Here's how the part is built. I have some questions about the finished solid (model axes, mm). Face numbers are marked on the shaded views. A direction names the side the tool comes from. Give positions to 0.01 mm unless a question says otherwise; leave off trailing zeros. Write each loop counter-clockwise with the first axis right and the second up, starting at its lowest first coordinate (ties: lowest second). Pieces come first, ordered by that corner, then holes. Notation, with made-up numbers: (56, 1) -> (74, 1) arc R22 cw to (74, 12) -> close; hole circle Ø7 at (49.5, -5). An arc over 180 degrees is marked (long way). Use one line per item in the form item = value.
```python
from build123d import *

# Parameters (mm, degrees)
F0_W      = 38.1
F0_H      = 38.1
F1_DEPTH  = 38.1
F2_T      = -2.54
F4_D      = 6.35
F5_R      = 1.55575
F7_DEPTH  = 35.56
F8_R      = 3.175
F9_R      = 3.175
F10_DEPTH = 38.101


with BuildPart() as f1:
    # F0 (on Top) → F1 (new body)
    with BuildSketch(Plane.XY):
        with Locations((8.3189541474, 5.4249440373)):
            Rectangle(F0_W, F0_H)
    extrude(amount=F1_DEPTH)

    # F2
    f2_openings = [f1.faces().sort_by_distance(p)[0] for p in [
        (8.318954, 5.424944, 38.1),
    ]]
    offset(amount=F2_T, openings=f2_openings)

    # F4 (through all)
    with Locations(Plane(origin=(0, 0, 0), x_dir=(1, 0, 0), z_dir=(0, 0, -1))):
        with Locations((8.3189541474, -5.4249440373)):
            Hole(F4_D / 2)

    # F5
    f5_edges = [f1.edges().sort_by_distance(p)[0] for p in [
        (8.318954, -13.625056, 0),
        (-10.731046, 5.424944, 0),
        (27.368954, 5.424944, 0),
        (8.318954, 24.474944, 0),
        (27.368954, 24.474944, 19.05),
        (27.368954, -13.625056, 19.05),
        (-10.731046, 24.474944, 19.05),
        (-10.731046, -13.625056, 19.05),
    ]]
    fillet(f5_edges, radius=F5_R)

    # F6 (on face) → F7 (join, through all)
    with BuildSketch(Plane.XY.offset(38.1)):
        with BuildLine():
            Line((24.8289541474, -11.0850559627), (24.8289541474, -6.3225559627))
            ThreePointArc((24.8289541474, -6.3225559627), (21.461358102, -7.7174599173), (20.0664541474, -11.0850559627))
            Line((20.0664541474, -11.0850559627), (24.8289541474, -11.0850559627))
        make_face()
        with BuildLine():
            Line((24.8289541474, 21.9349440373), (20.3255117221, 21.9349440373))
            ThreePointArc((20.3255117221, 21.9349440373), (21.6370716814, 18.6732811952), (24.8289541474, 17.2000126029))
            Line((24.8289541474, 17.2000126029), (24.8289541474, 21.9349440373))
        make_face()
        with BuildLine():
            Line((-8.1910458526, 21.9349440373), (-8.1910458526, 17.2900056063))
            ThreePointArc((-8.1910458526, 17.2900056063), (-4.797077777, 18.606071813), (-3.3241014455, 21.9349440373))
            Line((-3.3241014455, 21.9349440373), (-8.1910458526, 21.9349440373))
        make_face()
        with BuildLine():
            Line((-8.1910458526, -11.0850559627), (-3.6057208911, -11.0850559627))
            ThreePointArc((-3.6057208911, -11.0850559627), (-4.9295289639, -7.7640913608), (-8.1910458526, -6.2999256305))
            Line((-8.1910458526, -6.2999256305), (-8.1910458526, -11.0850559627))
        make_face()
    extrude(amount=-F7_DEPTH)

    # F8
    f8_edges = [f1.edges().sort_by_distance(p)[0] for p in [
        (24.828954, 17.200013, 20.32),
        (24.828954, 5.438728, 2.54),
        (21.637072, 18.673281, 2.54),
        (20.325512, 21.934944, 20.32),
        (8.500705, 21.934944, 2.54),
        (24.828954, -6.322556, 20.32),
        (21.461358, -7.71746, 2.54),
        (20.066454, -11.085056, 20.32),
        (8.230367, -11.085056, 2.54),
        (-4.929529, -7.764091, 2.54),
        (-8.191046, -6.299926, 20.32),
        (-3.605721, -11.085056, 20.32),
        (-4.797078, 18.606072, 2.54),
        (-8.191046, 17.290006, 20.32),
        (-8.191046, 5.49504, 2.54),
        (-3.324101, 21.934944, 20.32),
    ]]
    fillet(f8_edges, radius=F8_R)

    # F9 (on face) → F10 (cut, through all)
    with BuildSketch(Plane(origin=(0, 0, 0), x_dir=(1, 0, 0), z_dir=(0, 0, -1))):
        with Locations((14.6689541474, 0.9250559627)):
            Circle(F9_R)
    extrude(amount=-F10_DEPTH, mode=Mode.SUBTRACT)


solid = f1.part
```
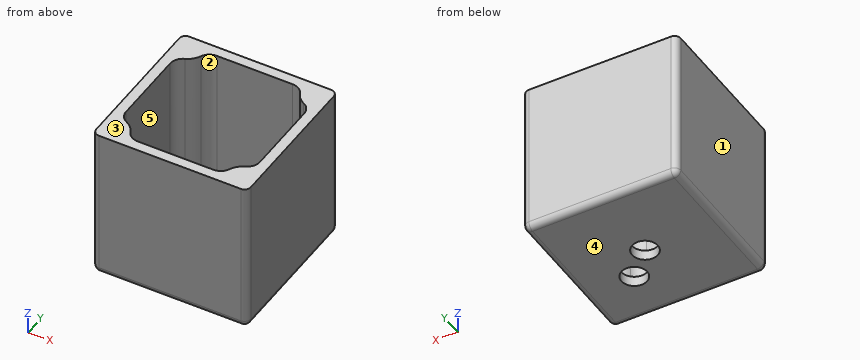
Q1. If we mould it in two halves opening along X, with no side actions, what happens to the marked faces 1, 2 and 3? For each: +X half, -X half, draft (parallel to the pull), parting line (faces both ways), or undercut.
Result set:
face_1 = -X half
face_2 = undercut
face_3 = draft
Q2. If I drill on line 1 along X through (y, z) = (10, 27); line 2 along Y through (x, z) = (17, 21.5); line 3 along X through (y, z) = (-6.5, 4), over which ranges is the centre line in solid material (lowest first)? Write a range as from..to.
Result set:
line_1 = -10.73..-8.19, 24.83..27.37
line_2 = -13.63..-11.09, 21.93..24.47
line_3 = -10.73..-5.73, 22.24..27.37
Q3. I want a section at D-D, the plane x = -7.5. Write out the boundary of the cut face in (y, z) (1 decimal), and give its area (3 significant figures).
Result set:
outline = (-13.6, 1.6) arc R1.6 ccw to (-12.1, 0) -> (22.9, 0) arc R1.6 ccw to (24.5, 1.6) -> (24.5, 38.1) -> (16.7, 38.1) -> (16.7, 5.7) arc R2 cw to (14.7, 3.7) -> (-3.9, 3.7) arc R2 cw to (-5.8, 5.7) -> (-5.8, 38.1) -> (-13.6, 38.1) -> close
area = 677 mm2
Q4. Will these pins go through, and if not, where does the flat tip stop? pin 1 Ø12 at (x, y) = (-1.5, 3.5) entering from +Z; pin 2 Ø13.5 at (x, y) = (7.5, 3.5) entering from +Z.
Result set:
pin_1 = 3.74
pin_2 = 2.54
Q5. Which directions (+Z, -Z, +X, -X, +Y, -Y) give clear straight access to the entire face, cutting with the end or side of a thin tool? Please do the marked faces 4 and 5.
Result set:
face_4 = -Z, +X, -X, +Y, -Y
face_5 = +Z
